The model under review builds one solid part; all positions refer to its coordinate system, in mm. A direction names the side the tool comes from. Round coordinates to 2 decimals unless told otherwise and drop trailing zeros. Order: outer loops, then holes, each group sorted by start corner. A loop starts at its lowest first (then second) coordinate and runs counter-clockwise, first axis right, second up. Notation, with made-up numbers: M 26,-39 L 36,-39 A16 ccw 36,-22 Z; hole C 55.5,78 d2. An arc over 180 degrees is marked long. Answer as a JSON object with one key per item and string values. Group by question number.
1. To check wall thickness, follow probe 1 along X at (y, z) = (0.45, -45); probe 2 along Y at (x, z) = (14.5, -46); probe 3 along Z at (x, y) = (11, 13). State the ranges of each line that lie inside material, in increasing order. Write a range as [from, to].
2. Add section A-A on x = 15. State the section outline as (y, z) points.
3. Machinability: for faces 1 (the face through (10.12, 59.51, -16.08)), 2 (the face through (49.995, 30.22, -59.507)), 3 (the face through (59.507, 10.564, -17.307)), 4 (the face through (1, 45, -45)), 5 (the face through (15, 1, -45)), which of the approach directions +Z, -Z, +X, -X, +Y, -Y give a long, thin tool a straight path to every point of the face, cutting with its end or side? Answer none if there is none.
4. Mouldability with a two-part tool opening along Y and no side actions: class faces 6 (the face through (25.005, 30.22, -0.493)), 7 (the face through (15, 59, -15)), 8 (the face through (23, 30, 0)) as released by +Y, released by -Y, zero draft, split by the parting line, or undercut.
5. Add section B-B on z = -45. State the section outline as (x, y) points, and give its area (3 significant figures).
6. Clearance check with flat-ended pins moving along their axes: P1, Ø3, axis at x = 46, y = 44.5, coming from the -Z side; P2, Ø5, axis at y = 17, z = -45.5, coming from the -X side; P3, Ø5, axis at y = 16, z = -15, coming from the +X side. State where each tip first meets the part, or that it passes through.
```python
from build123d import *

# Parameters (mm, degrees)
SKETCH1_W          = 60
SKETCH1_H          = 60
EXTRUDE1_DEPTH     = 60
SKETCH2_R          = 5
CUT_EXTRUDE1_DEPTH = 1
SKETCH3_R          = 5
CUT_EXTRUDE2_DEPTH = 1
SKETCH4_R          = 5
CUT_EXTRUDE3_DEPTH = 1
SKETCH5_R          = 5
CUT_EXTRUDE4_DEPTH = 1
SKETCH6_R          = 5
CUT_EXTRUDE5_DEPTH = 1
SKETCH7_R          = 5
CUT_EXTRUDE6_DEPTH = 1


with BuildPart() as part:
    # Sketch1 → Extrude1 (new body)
    with BuildSketch(Plane(origin=(0, 0, 0), x_dir=(1, 0, 0), z_dir=(0, 1, 0))):
        with Locations((30, 30)):
            Rectangle(SKETCH1_W, SKETCH1_H)
    extrude(amount=EXTRUDE1_DEPTH)

    # Sketch2 → Cut-Extrude1 (cut)
    with BuildSketch(Plane(origin=(0, 60, 0), x_dir=(-1, 0, 0), z_dir=(0, 1, 0))):
        with Locations(Location((-45, -45, 0), (0, 0, 90))):  # turned: the seam where the file's is
            Circle(SKETCH2_R)
        with Locations(Location((-30, -30, 0), (0, 0, 90))):  # turned: the seam where the file's is
            Circle(SKETCH2_R)
        with Locations(Location((-15, -15, 0), (0, 0, 90))):  # turned: the seam where the file's is
            Circle(SKETCH2_R)
    extrude(amount=-CUT_EXTRUDE1_DEPTH, mode=Mode.SUBTRACT)

    # Sketch3 → Cut-Extrude2 (cut)
    with BuildSketch(Plane(origin=(60, 0, 0), x_dir=(0, 0, -1), z_dir=(1, 0, 0))):
        with Locations((45, 45)):
            Circle(SKETCH3_R)
        with Locations((15, 15)):
            Circle(SKETCH3_R)
    extrude(amount=-CUT_EXTRUDE2_DEPTH, mode=Mode.SUBTRACT)

    # Sketch4 → Cut-Extrude3 (cut)
    with BuildSketch(Plane.XY):
        with Locations((30, 30)):
            Circle(SKETCH4_R)
    extrude(amount=-CUT_EXTRUDE3_DEPTH, mode=Mode.SUBTRACT)

    # Sketch5 → Cut-Extrude4 (cut)
    with BuildSketch(Plane(origin=(0, 0, -60), x_dir=(-1, 0, 0), z_dir=(0, 0, -1))):
        with Locations((-15, 45)):
            Circle(SKETCH5_R)
        with Locations((-15, 30)):
            Circle(SKETCH5_R)
        with Locations((-15, 15)):
            Circle(SKETCH5_R)
        with Locations((-45, 45)):
            Circle(SKETCH5_R)
        with Locations((-45, 30)):
            Circle(SKETCH5_R)
        with Locations((-45, 15)):
            Circle(SKETCH5_R)
    extrude(amount=-CUT_EXTRUDE4_DEPTH, mode=Mode.SUBTRACT)

    # Sketch6 → Cut-Extrude5 (cut)
    with BuildSketch(Plane.ZY):
        with Locations((-30, 30)):
            Circle(SKETCH6_R)
        with Locations(Location((-45, 45, 0), (0, 0, 180))):  # turned: the seam where the file's is
            Circle(SKETCH6_R)
        with Locations((-15, 45)):
            Circle(SKETCH6_R)
        with Locations((-45, 15)):
            Circle(SKETCH6_R)
        with Locations(Location((-15, 15, 0), (0, 0, 180))):  # turned: the seam where the file's is
            Circle(SKETCH6_R)
    extrude(amount=-CUT_EXTRUDE5_DEPTH, mode=Mode.SUBTRACT)

    # Sketch7 → Cut-Extrude6 (cut)
    with BuildSketch(Plane.XZ):
        with Locations(Location((15, -45, 0), (0, 0, 270))):  # turned: the seam where the file's is
            Circle(SKETCH7_R)
        with Locations(Location((15, -15, 0), (0, 0, 90))):  # turned: the seam where the file's is
            Circle(SKETCH7_R)
        with Locations(Location((45, -45, 0), (0, 0, 90))):  # turned: the seam where the file's is
            Circle(SKETCH7_R)
        with Locations(Location((45, -15, 0), (0, 0, 270))):  # turned: the seam where the file's is
            Circle(SKETCH7_R)
    extrude(amount=-CUT_EXTRUDE6_DEPTH, mode=Mode.SUBTRACT)


solid = part.part
```
Recorded:
{
 "1": {"probe 1": "x = [0, 10], [20, 40], [50, 60]", "probe 2": "y = [1, 60]", "probe 3": "z = [-59, 0]"},
 "2": {"outline": "M 0,-60 L 10,-60 L 10,-59 L 20,-59 L 20,-60 L 25,-60 L 25,-59 L 35,-59 L 35,-60 L 40,-60 L 40,-59 L 50,-59 L 50,-60 L 60,-60 L 60,-20 L 59,-20 L 59,-10 L 60,-10 L 60,0 L 0,0 L 0,-10 L 1,-10 L 1,-20 L 0,-20 L 0,-40 L 1,-40 L 1,-50 L 0,-50 Z"},
 "3": {"face 1": "+Y", "face 2": "-Z", "face 3": "+X", "face 4": "-X", "face 5": "-Y"},
 "4": {"face 6": "undercut", "face 7": "released by +Y", "face 8": "zero draft"},
 "5": {"outline": "M 0,0 L 10,0 L 10,1 L 20,1 L 20,0 L 40,0 L 40,1 L 50,1 L 50,0 L 60,0 L 60,40 L 59,40 L 59,50 L 60,50 L 60,60 L 50,60 L 50,59 L 40,59 L 40,60 L 0,60 L 0,50 L 1,50 L 1,40 L 0,40 L 0,20 L 1,20 L 1,10 L 0,10 Z", "area": "3,540 mm²"},
 "6": {"P1": "stops at z = -59", "P2": "stops at x = 1", "P3": "stops at x = 59"}
}
